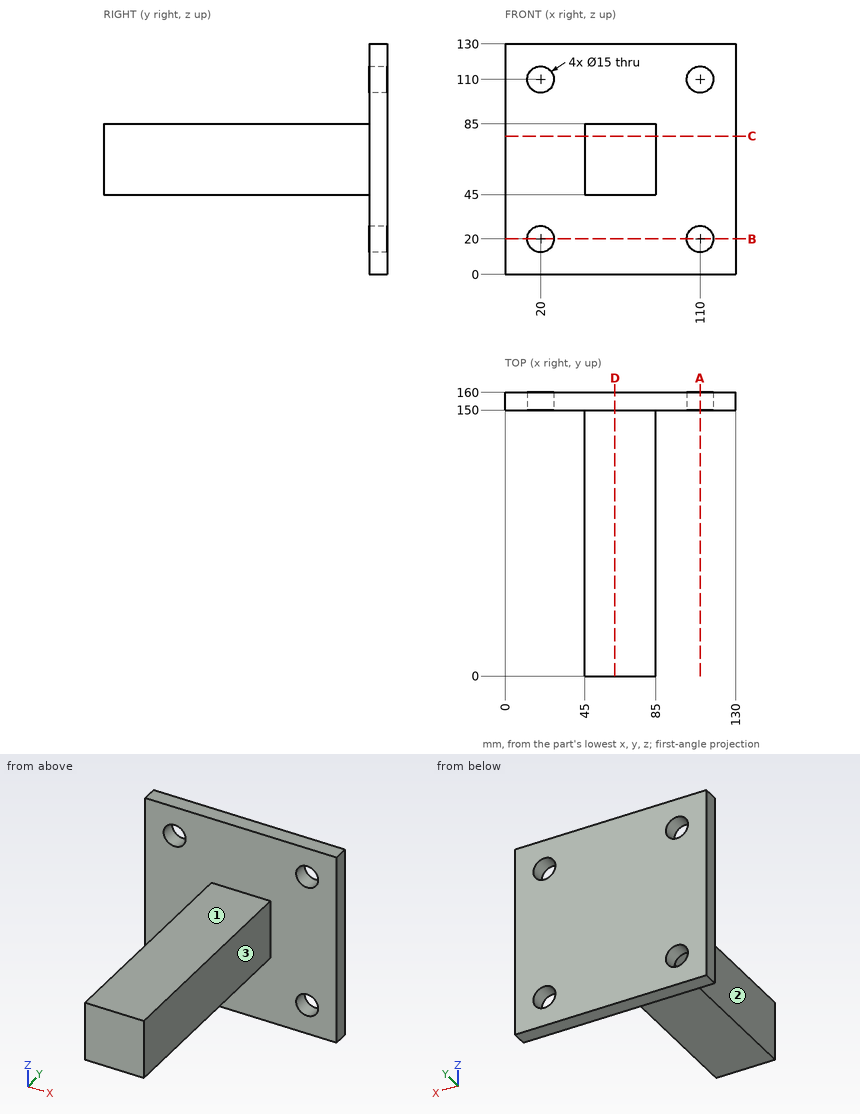
Study the drawing (mm; zero at the part's minimum x, y, z) and answer. A direction names the side the tool comes from. Give positions to 0.01 mm unless a question says otherwise; leave off trailing zeros. Loops run counter-clockwise (first coordinate to the right, second up) from the corner with the lowest first, then second, coordinate; pieces in that order, holes last. Notation, with made-up numbers: (28, 15) - (59, 15) arc R20 ccw to (59, 33) - close; hole circle Ø1 at (79.5, 26.25). An arc over 180 degrees is marked (long way). Answer as CSV lines item,"result". Start each with the question number.
1) Find section B-B (z = 20). Write down the section's boundary in (x, y).
2) Find section A-A (x = 110). Write down the section's boundary in (y, z).
3) Each of these flat-tipped pins is pushed along its axis until it touches: pin 1 Ø12 at (x, y) = (67.5, 62) entering from +Z; pin 2 Ø2 at (x, z) = (60.5, 26.5) entering from -Y; pin 3 Ø12 at (y, z) = (45, 59) entering from +X. Where does it stop, or does it pass through?
4) Straight lines are drawn through the part: L1, parallel to X at y = 154.25, z = 110; L2, parallel to Y at x = 8.5, z = 123.5; L3, parallel to X at y = 15, z = 83. For each, find the intervals that lie inside material, in ascending order. Write a range as from..to.
5) Find section C-C (z = 78). Write down the section's boundary in (x, y).
6) Find section D-D (x = 62). Write down the section's boundary in (y, z).
7) Which of the six approach directions +Z, -Z, +X, -X, +Y, -Y give full straight-line access (tool end or side, diameter ignored) to the marked faces 1, 2 and 3?
Findings below:
1,outline,"(0, 150) - (12.5, 150) - (12.5, 160) - (0, 160) - close; (27.5, 150) - (102.5, 150) - (102.5, 160) - (27.5, 160) - close; (117.5, 150) - (130, 150) - (130, 160) - (117.5, 160) - close"
2,outline,"(150, 0) - (160, 0) - (160, 12.5) - (150, 12.5) - close; (150, 27.5) - (160, 27.5) - (160, 102.5) - (150, 102.5) - close; (150, 117.5) - (160, 117.5) - (160, 130) - (150, 130) - close"
3,pin 1,"z = 85"
3,pin 2,"y = 150"
3,pin 3,"x = 85"
4,L1,"0..12.5, 27.5..102.5, 117.5..130"
4,L2,"150..160"
4,L3,"45..85"
5,outline,"(0, 150) - (45, 150) - (45, 0) - (85, 0) - (85, 150) - (130, 150) - (130, 160) - (0, 160) - close"
6,outline,"(0, 45) - (150, 45) - (150, 0) - (160, 0) - (160, 130) - (150, 130) - (150, 85) - (0, 85) - close"
7,face 1,"+Z, +X, -X, -Y"
7,face 2,"+Z, -Z, -X, -Y"
7,face 3,"+Z, -Z, +X, -Y"
